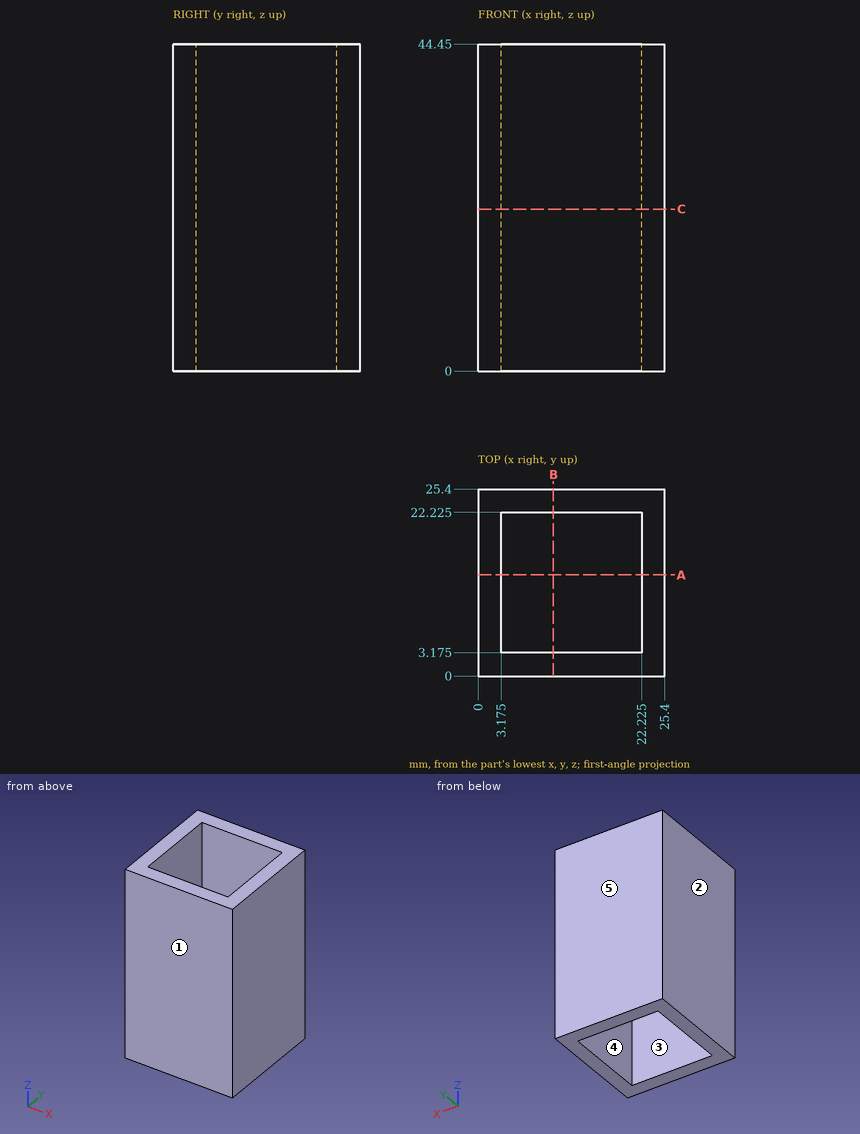
Verification items for this drawing (mm, ordinates from the low corner). A direction names the side the tool comes from. Coordinates: 2 decimals unless noted, no trailing zeros. Order: outer loops, then holes, each group sorted by start corner. A loop starts at its lowest first (then second) coordinate and runs counter-clockwise, first axis right, second up. Notation, with made-up numbers: M 6.5,81 L 21.5,81 A33 ccw 21.5,117 Z; hole C 38.25,-19.75 d2. An arc over 180 degrees is marked long. Answer as a JSON object with one key per item and string values.
Q1. Scan line: line 1 (X direction, y = 14, z = 36.5) (3 decimals). Record every from-to range of solid material in increasing order.
Results are:
{"line 1": "x = 0 to 3.175, 22.225 to 25.4"}
Q2. Release check for a two-part mould opening along Y. For the marked faces 1, 2 and 3 record: released by +Y, released by -Y, zero draft, split by the parting line, or undercut.
Results are:
{"face 1": "released by -Y", "face 2": "zero draft", "face 3": "undercut"}
Q3. Depth check by flat-ended pin: pin 1 Ø1.5 at (y, z) = (9.5, 34) entering from -X. Enter the tip coordinate at first touch or a pass-through.
Results are:
{"pin 1": "stops at x = 0"}
Q4. Cross-section at C-C on z = 22. Record the cut outline in (x, y) (3 decimals).
Results are:
{"outline": "M 0,0 L 25.4,0 L 25.4,25.4 L 0,25.4 Z; hole M 3.175,3.175 L 22.225,3.175 L 22.225,22.225 L 3.175,22.225 Z"}
Q5. Tool access check on the marked faces 4 and 5. Record the directions out of +Z, -Z, +X, -X, +Y, -Y that give a thin tool (end or side, any length) a straight path to the whole face; none if there is none.
Results are:
{"face 4": "+Z, -Z", "face 5": "+Z, -Z, +X, -X, +Y"}
Q6. Cross-section at A-A on y = 13.75. Record the cut outline in (x, z) (3 decimals).
Results are:
{"outline": "M 0,0 L 3.175,0 L 3.175,44.45 L 0,44.45 Z; M 22.225,0 L 25.4,0 L 25.4,44.45 L 22.225,44.45 Z"}
